Read the model definition and answer for the solid it produces. Units are mm, in the model's axes. A direction names the side the tool comes from. Round coordinates to 2 decimals unless told otherwise and drop trailing zeros. Order: outer loops, then holes, each group sorted by start corner. A loop starts at its lowest first (then second) coordinate and runs counter-clockwise, first axis right, second up. Notation, with made-up numbers: (-5, 81.5) -> (34, 81.5) arc R25 ccw to (34, 120.5) -> close; hole circle Ø3 at (60, 62). An arc over 180 degrees is marked (long way). Answer as a JSON object with one key per item and string values. Group by question number.
Item 1: Section A-A, the plane x = 50 is taken. Write down the section's boundary in (y, z), plus the area to 3 significant figures.
Item 2: Section D-D, the plane y = -5 is taken. Write down the section's boundary in (x, z), plus the area to 3 significant figures.
Item 3: Given P1, Ø1.5, axis at x = 49.5, z = -1, coming from the -Y side, flat-ended and moving along its own axis, determine where the tip first touches the part or whether it passes through.
Item 4: Consider probe 1 along X at (y, z) = (1.5, -0.95); probe 2 along Y at (x, z) = (65, -2.1); probe 3 along Y at (x, z) = (60, -0.65). Determine where each line is inside the solid, lowest interval first. Write a range as from..to.
Item 5: Section B-B, the plane z = -0.75 is taken. Write down the section's boundary in (x, y).
Item 6: The mould has two halves that part along Y. Classify faces 3 (the flat face through (75, 0, -1)), 4 (the cylindrical face through (67.68, -1.11, -1.52)), 5 (the flat face through (-14.76, -38.05, -1.48)): pulls with the +Y half, pulls with the -Y half, needs draft (parallel to the pull), parting line crosses it, or undercut.
Item 7: For faces 1 (the flat face through (39, -10, -1)), 2 (the cylindrical face through (74.14, 9.1, -1.48)), determine the directions among +Z, -Z, +X, -X, +Y, -Y from which every point of the face is accessible in a straight line to the end or side of a thin tool.
Item 8: Section C-C, the plane x = 31.5 is taken. Write down the section's boundary in (y, z), plus the area to 3 significant figures.
from build123d import *

# Parameters (mm, degrees)
BOSS_EXTRU_1_DEPTH       = 3
D_GAGEMENT_START         = -3
D_GAGEMENT_M51_OUTLINE_R = 2.9
D_GAGEMENT_M51_DEPTH     = 3


# Read off the part's stored shape, not the designer's step: Dégagement M51
with BuildPart() as part:
    # Esquisse1 → Boss.-Extru.1 (new body)
    with BuildSketch(Plane.XY):
        with BuildLine():
            Line((-6.724255553, 8.256356511), (-38.711792489, -61.104708083))
            ThreePointArc((-38.711792489, -61.104708083), (-37.5, -64.951905284), (-33.554116714, -64.115620384))
            Line((-33.554116714, -64.115620384), (4.566579778, -11.24544421))
            ThreePointArc((4.566579778, -11.24544421), (5.633191193, -10.329450677), (7, -10))
            Line((7, -10), (72, -10))
            ThreePointArc((72, -10), (74.121320344, -9.121320344), (75, -7))
            Line((75, -7), (75, 7))
            ThreePointArc((75, 7), (74.121320344, 9.121320344), (72, 10))
            Line((72, 10), (-4, 10))
            ThreePointArc((-4, 10), (-5.617240005, 9.526763694), (-6.724255553, 8.256356511))
        make_face()
    extrude(amount=-BOSS_EXTRU_1_DEPTH)

    # Dégagement M51 outline → Dégagement M51 (cut)
    with BuildSketch(Plane.XY.offset(D_GAGEMENT_START)):
        with Locations((65, 0)):
            Circle(D_GAGEMENT_M51_OUTLINE_R)
        with Locations((50, 0)):
            Circle(D_GAGEMENT_M51_OUTLINE_R)
        with Locations((-15, -25.980762114)):
            Circle(D_GAGEMENT_M51_OUTLINE_R)
        with Locations((30, 0)):
            Circle(D_GAGEMENT_M51_OUTLINE_R)
    extrude(amount=D_GAGEMENT_M51_DEPTH, mode=Mode.SUBTRACT)


solid = part.part
Values found:
{
 "1": {"outline": "(-10, -3) -> (-2.9, -3) -> (-2.9, 0) -> (-10, 0) -> close; (2.9, -3) -> (10, -3) -> (10, 0) -> (2.9, 0) -> close", "area": "42.6 mm2"},
 "2": {"outline": "(-12.84, -3) -> (75, -3) -> (75, 0) -> (-12.84, 0) -> close", "area": "264 mm2"},
 "3": {"P1": "y = -10"},
 "4": {"probe 1": "-9.84..27.52, 32.48..47.52, 52.48..62.52, 67.48..75", "probe 2": "-10..-2.9, 2.9..10", "probe 3": "-10..10"},
 "5": {"outline": "(-38.71, -61.1) arc R3 ccw to (-33.55, -64.12) -> (4.57, -11.25) arc R3 cw to (7, -10) -> (72, -10) arc R3 ccw to (75, -7) -> (75, 7) arc R3 ccw to (72, 10) -> (-4, 10) arc R3 ccw to (-6.72, 8.26) -> close; hole circle Ø5.8 at (-15, -25.98); hole circle Ø5.8 at (30, 0); hole circle Ø5.8 at (50, 0); hole circle Ø5.8 at (65, 0)"},
 "6": {"face 3": "needs draft", "face 4": "undercut", "face 5": "pulls with the -Y half"},
 "7": {"face 1": "+Z, -Z, +X, -Y", "face 2": "+Z, -Z, +X, +Y"},
 "8": {"outline": "(-10, -3) -> (-2.48, -3) -> (-2.48, 0) -> (-10, 0) -> close; (2.48, -3) -> (10, -3) -> (10, 0) -> (2.48, 0) -> close", "area": "45.1 mm2"}
}
